Autodesk Inventor part; units mm, degrees
ref_plane "YZ Plane" through (0, 0, 0) normal (1, 0, 0) x (0, 1, 0)
ref_plane "XZ Plane" through (0, 0, 0) normal (0, 1, 0) x (-1, 0, 0)
ref_plane "XY Plane" through (0, 0, 0) normal (0, 0, 1) x (1, 0, 0)
sketch "Sketch1" plane through (0, 0, 0) normal (0, 0, 1) x (1, 0, 0)
  line L0 (355.6, 50.8) -> (-19.05, 50.8)
  line L1 (12.7, 50.8) -> (12.7, 0) construction
  line L2 (0, 38.1) -> (12.7, 38.1) construction
  line L3 (0, 12.7) -> (12.7, 12.7) construction
  circle A0 centre (12.7, 38.1) radius 3.175
  circle A1 centre (12.7, 12.7) radius 3.175
  line L4 (168.275, 50.8) -> (168.275, 0) construction
  line L5 (-19.05, 50.8) -> (-19.05, 0)
  line L6 (355.6, 50.8) -> (355.6, 0)
  circle A2 centre (-9.525, 25.4) radius 3.175
  circle A3 centre (323.85, 38.1) radius 3.175
  circle A4 centre (323.85, 12.7) radius 3.175
  line L7 (355.6, 50.8) -> (355.6, 0)
  circle A5 centre (346.075, 25.4) radius 3.175
  line L8 (-19.05, 0) -> (355.6, 0)
  dimension "d0" = 374.65
  dimension "d3" = 12.7
  dimension "d4" = 25.4
  dimension "d5" = 6.35
  dimension "d6" = 6.35
  dimension "d10" = 6.35
  dimension "d11" = 31.75
extrude "Extrusion2" add sketch "Sketch1" along normal blind 3.175
sketch "Sketch3" plane through (0, 0, 3.175) normal (0, 0, 1) x (1, 0, 0)
  line L0 (-19.05, 50.8) -> (-19.05, 0)
  line L1 (-19.05, 25.4) -> (168.275, 25.4)
  line L2 (355.6, 50.8) -> (-19.05, 50.8)
  line L3 (168.275, 25.4) -> (168.275, 50.8)
  point P0 (0, 0)
hole "Hole1" at (168.275, 25.4, 3.175) direction (0, 0, -1) diameter 22.86 depth 25.4 tip angle 118
sketch "Sketch4" plane through (0, 0, 3.175) normal (0, 0, 1) x (1, 0, 0)
  circle A0 centre (168.275, 25.4) radius 11.43
  line L0 (168.275, 25.4) -> (142.875, 25.4)
  circle A1 centre (142.875, 25.4) radius 3.175
  line L1 (355.6, 50.8) -> (-19.05, 50.8)
  line L2 (168.275, 50.8) -> (168.275, 0)
  circle A2 centre (193.675, 25.4) radius 3.175
  point P0 (0, 0)
  dimension "d21" = 25.4
  dimension "d22" = 6.35
hole "Hole2" at (193.675, 25.4, 3.175) at (142.875, 25.4, 3.175) direction (0, 0, -1) diameter 6.35 depth 25.4 tip angle 118
sketch "Sketch5" plane through (0, 0, 3.175) normal (0, 0, 1) x (1, 0, 0)
  line L0 (355.6, 50.8) -> (-19.05, 50.8)
  line L1 (74.6506, 50.8) -> (74.6506, 0)
  line L2 (-19.05, 50.8) -> (-19.05, 0)
  line L3 (74.6506, 50.8) -> (74.6506, 44.45)
  line L4 (74.6506, 44.45) -> (74.6506, 25.4)
  circle A0 centre (74.6506, 44.45) radius 2.0701
  line L5 (74.6506, 25.4) -> (74.6506, 6.35)
  circle A1 centre (74.6506, 25.4) radius 2.0701
  circle A2 centre (74.6506, 6.35) radius 2.0701
  line L6 (168.275, 50.8) -> (168.275, 0)
  circle A3 centre (261.8994, 44.45) radius 2.0701
  circle A4 centre (261.8994, 25.4) radius 2.0701
  circle A5 centre (261.8994, 6.35) radius 2.0701
  point P0 (0, 0)
  dimension "d30" = 93.7006
  dimension "d31" = 6.35
  dimension "d32" = 19.05
  dimension "d33" = 4.1402
  dimension "d34" = 19.05
  dimension "d35" = 4.1402
  dimension "d36" = 4.1402
hole "Hole3" at (74.6506, 44.45, 3.175) at (74.6506, 25.4, 3.175) at (74.6506, 6.35, 3.175) at (261.8994, 44.45, 3.175) at (261.8994, 25.4, 3.175) at (261.8994, 6.35, 3.175) direction (0, 0, -1) diameter 4.1402 depth 25.4 tip angle 118
sketch "Sketch6" plane through (0, 0, 3.175) normal (0, 0, 1) x (1, 0, 0)
  circle A0 centre (12.7, 38.1) radius 3.175
  line L0 (12.7, 38.1) -> (25.4, 38.1)
  line L1 (355.6, 50.8) -> (-19.05, 50.8)
  line L2 (25.4, 50.8) -> (25.4, 0)
  point P0 (0, 0)
  dimension "d44" = 12.7
split body "Split1" sketch "Sketch6" result one side removed curves L2 removed pieces at (41.1319, 25.4832, 0.5)
properties part number "2AM-17-P-0206 - moving support slider panl" material "Aluminum 6061"
Can you work these out from the model? Positions are in its coordinate system, mm. Coordinates: 2 decimals unless noted, no trailing zeros. Loops run counter-clockwise (first coordinate to the right, second up) from the corner with the lowest first, then second, coordinate; pieces in that order, holes last. Notation, with made-up numbers: M 59,62.25 L 115,62.25 A25 ccw 115,95.25 Z; hole C 28.25,53.25 d1. An arc over 180 degrees is marked long. Return JSON: item names as keys, results as strings. Group by question number.
Item 1: Thinking about a two-plate mould opening in Y: for faces 1 (the cylindrical face through (10.18, 14.63, 1.57)), 2 (the cylindrical face through (12.29, 34.95, 1.57)), 3 (the flat face through (3, 26, 0)), 4 (the flat face through (3, 0, 2)), which applies, released by +Y, released by -Y, zero draft, split by the parting line, or undercut?
Item 2: Imagine slicing it at A-A (x = 12.7). Please give me the cut outline in (y, z) (3 decimals).
Item 3: Imagine slicing it at B-B (y = 12.7). Please give me the cut outline in (x, z) (3 decimals).
Item 4: I'm going to push a flat-ended pin straight in: pin 1 Ø5 at (x, y) = (12.7, 12.7) entering from -Z. Where does the tip first touch, or does it pass through?
Item 5: If I drill on L1, parallel to Y at x = 12.7, z = 1.3 (3 decimals); L2, parallel to Y at x = 13.5, z = 0.1; L3, parallel to X at y = 13, z = 0.6, over which ranges is the centre line in solid material (lowest first)? Write a range as from..to.
Verdict:
{
 "1": {"face 1": "undercut", "face 2": "undercut", "face 3": "zero draft", "face 4": "released by -Y"},
 "2": {"outline": "M 0,0 L 9.525,0 L 9.525,3.175 L 0,3.175 Z; M 15.875,0 L 34.925,0 L 34.925,3.175 L 15.875,3.175 Z; M 41.275,0 L 50.8,0 L 50.8,3.175 L 41.275,3.175 Z"},
 "3": {"outline": "M -19.05,0 L 9.525,0 L 9.525,3.175 L -19.05,3.175 Z; M 15.875,0 L 25.4,0 L 25.4,3.175 L 15.875,3.175 Z"},
 "4": {"pin 1": "passes through"},
 "5": {"L1": "y = 0..9.525, 15.875..34.925, 41.275..50.8", "L2": "y = 0..9.63, 15.77..35.03, 41.17..50.8", "L3": "x = -19.05..9.54, 15.86..25.4"}
}
